Input: part model. Units: mm. Frame: model coordinates. Give positions to 0.01 mm unless a question says otherwise; leave off trailing zeros. Loops run counter-clockwise (first coordinate to the right, second up) from the corner with the lowest first, then second, coordinate; pieces in that order, holes last. Notation, with made-up numbers: M 36,82.25 L 83,82.25 A27 ccw 83,112.25 Z; hole C 83,20 d5. An arc over 180 degrees is marked long. Answer as a JSON object with one key per item and string values. Group by question number.
1) Section query A-A on y = 5.5. Return loops of the section in (x, z), plus the area to 3 significant figures.
2) Section query D-D on z = 0.6. Return loops of the section in (x, y).
3) Section query C-C on x = 1.5. Return loops of the section in (y, z).
4) Section query B-B on x = 23. Return loops of the section in (y, z), plus the area to 3 significant figures.
5) Ray query, L1, parallel to Y at x = 23, z = 4.85; L2, parallel to Y at x = 22, z = 5.4; L3, parallel to X at y = -5.5, z = 1.55. Return the intervals inside material, ascending.
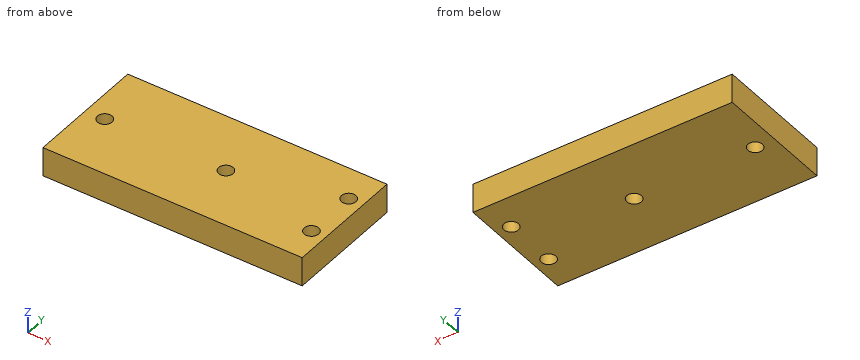
from build123d import *

# Parameters (mm, degrees)
F0_W     = 55
F0_H     = 25
F1_DEPTH = 6
F2_D     = 3
F3_DEPTH = 1.5


# Not quite as in the source:
# - a feature names something its author has since deleted; it is built from what else it names


with BuildPart() as f1:
    # F0 (on Top) → F1 (new body)
    with BuildSketch(Plane.XY):
        Rectangle(F0_W, F0_H)
    extrude(amount=F1_DEPTH)

    # F2 (through all)
    with Locations(Plane(origin=(0, 0, 0), x_dir=(1, 0, 0), z_dir=(0, 0, -1))):
        with Locations((-23.5, 0), (23, -5.5), (23, 5.5), (1.5, 0)):
            Hole(F2_D / 2)

    # F3 (cut): a face of the model
    f3_faces = [f1.faces().sort_by_distance(p)[0] for p in [
        (27.5, 0, 3),
    ]]
    extrude(f3_faces, amount=-F3_DEPTH, mode=Mode.SUBTRACT)


solid = f1.part
Output:
{
 "1": {"outline": "M -27.5,0 L 21.5,0 L 21.5,6 L -27.5,6 Z; M 24.5,0 L 26,0 L 26,6 L 24.5,6 Z", "area": "303 mm^2"},
 "2": {"outline": "M -27.5,-12.5 L 26,-12.5 L 26,12.5 L -27.5,12.5 Z; hole C -23.5,0 d3; hole C 1.5,0 d3; hole C 23,-5.5 d3; hole C 23,5.5 d3"},
 "3": {"outline": "M -12.5,0 L -1.5,0 L -1.5,6 L -12.5,6 Z; M 1.5,0 L 12.5,0 L 12.5,6 L 1.5,6 Z"},
 "4": {"outline": "M -12.5,0 L -7,0 L -7,6 L -12.5,6 Z; M -4,0 L 4,0 L 4,6 L -4,6 Z; M 7,0 L 12.5,0 L 12.5,6 L 7,6 Z", "area": "114 mm^2"},
 "5": {"L1": "y = -12.5 to -7, -4 to 4, 7 to 12.5", "L2": "y = -12.5 to -6.62, -4.38 to 4.38, 6.62 to 12.5", "L3": "x = -27.5 to 21.5, 24.5 to 26"}
}
